```python
from build123d import *

# Parameters (mm, degrees)
EXTRUDE_1_DEPTH         = 8
SKETCH_3_OUTSIDE_W      = 189.666
SKETCH_3_OUTSIDE_H      = 189.666
SKETCH_3_OUTSIDE_R      = 12
CUT_EXTRUDE_1_DEPTH     = 41.024992192
CUT_EXTRUDE_1_DRAFT     = -60
HOLE_WIZARD_M30_1_D     = 26.5
HOLE_WIZARD_M30_1_DEPTH = 10
CHAMFER_1_SIZE          = 1
CHAMFER_2_SIZE          = 1


with BuildPart() as part:
    # 草图1 → 凸台-拉伸1 (new body)
    with BuildSketch(Plane.XY):
        Polygon((0, 13.856406461), (-12, 6.92820323), (-12, -6.92820323), (0, -13.856406461), (12, -6.92820323), (12, 6.92820323), align=None)
    extrude(amount=-EXTRUDE_1_DEPTH)

    # 草图2 → 旋转1 (revolve)
    with BuildSketch(Plane(origin=(0, 0, 0), x_dir=(0, 0, -1), z_dir=(1, 0, 0))):
        Polygon((8, 0), (8, 13.856406461), (11.143593539, 17), (32, 17), (32, 0), align=None)
    revolve(axis=Axis((0, 0, -32), (0, 0, 1)))


with BuildPart() as cut_extrude_1_tool:
    # 草图3 outside → 切除-拉伸1 (with draft: the straight prism first)
    with BuildSketch(Plane.XY):
        Rectangle(SKETCH_3_OUTSIDE_W, SKETCH_3_OUTSIDE_H)
        Circle(SKETCH_3_OUTSIDE_R, mode=Mode.SUBTRACT)
    extrude(amount=-CUT_EXTRUDE_1_DEPTH)
    # 切除-拉伸1: the draft: its side faces are tilted about the plane it starts from
    cut_extrude_1_sides = [cut_extrude_1_tool.faces().sort_by_distance(p)[0] for p in [
        (0, -94.833, -20.512496096),
        (94.833, 0, -20.512496096),
        (0, 94.833, -20.512496096),
        (-94.833, 0, -20.512496096),
        (-12, 0, -20.512496096),
    ]]
    draft(cut_extrude_1_sides, Plane.XY, CUT_EXTRUDE_1_DRAFT)


with BuildPart() as part_1:
    add(part.part)

    # 切除-拉伸1: cut by cut_extrude_1_tool
    add(cut_extrude_1_tool.part, mode=Mode.SUBTRACT)

    # 草图4 → 切除-旋转1 (revolve, cut)
    with BuildSketch(Plane(origin=(0, 0, 0), x_dir=(0, 0, -1), z_dir=(1, 0, 0)), mode=Mode.PRIVATE) as cut_revolve_1_sk:
        Polygon((0, 0), (0, -7), (6, -7), (6, -9), (14, -9), (14, -14), (15, -14), (15, -15), (22, -15), (22, 0), align=None)
    revolve(cut_revolve_1_sk.sketch.rotate(Axis((0, 0, -22), (0, 0, 1)), 270), axis=Axis((0, 0, -22), (0, 0, 1)), mode=Mode.SUBTRACT)

    # M30 螺纹孔1
    with Locations(Plane(origin=(0, 0, -32), x_dir=(-1, 0, 0), z_dir=(0, 0, -1))):
        with Locations((0, 0)):
            Hole(HOLE_WIZARD_M30_1_D / 2, depth=HOLE_WIZARD_M30_1_DEPTH)

    # 倒角1
    chamfer_1_edges = [part_1.edges().sort_by_distance(p)[0] for p in [
        (0, -17, -32),
    ]]
    chamfer(chamfer_1_edges, length=CHAMFER_1_SIZE)

    # 倒角2
    chamfer_2_edges = [part_1.edges().sort_by_distance(p)[0] for p in [
        (7, 0, 0),
        (9, 0, -14),
    ]]
    chamfer(chamfer_2_edges, length=CHAMFER_2_SIZE)


solid = part_1.part
```
Build history of the part. All positions in model axes, mm. A direction names the side the tool comes from. Coordinates: 2 decimals unless noted, no trailing zeros. Order: outer loops, then holes, each group sorted by start corner. A loop starts at its lowest first (then second) coordinate and runs counter-clockwise, first axis right, second up. Notation, with made-up numbers: M -16,77 L 17,77 A14 ccw 17,81 Z; hole C 30,-0.5 d4. An arc over 180 degrees is marked long. One line per question, with ' | ' between items. Start each with the question number.
1. Mould opens along X. For faces 4 (the face through (1.517, 6.834, -3.535)), 5 (the face through (10.76, -6.248, -0.256)), 6 (the face through (0.03, 12.443, -0.256)) say: +X half, -X half, draft (parallel to the pull), parting line (faces both ways), or undercut.
2. Cut at A-A (z = -21). Write the cut outline in (x, y), plus the area to 3 significant figures.
3. Wall check: line 1 along Y through (x, z) = (0, -3.1); line 2 along Y through (x, z) = (0, -14.45); line 3 along Z through (x, y) = (5.5, 11). Give the ranges that are in metal, low to high. Write a range as [from, to].
4. Tool access for faces 1 (the face through (-6, 11, -8)), 2 (the face through (-6.084, -10.344, -3.944)), 3 (the face through (5.92, -10.44, -3.94)): list every direction of +Z, -Z, +X, -X, +Y, -Y with a clear straight run to the whole face (end or side of a thin tool).
5. Cut at B-B (z = -8.5). Write the cut outline in (x, y), plus the area to 3 significant figures.
6. Flat gauge pins, fed straight in: P1, Ø8, axis at y = 3, z = -20, coming from the -X side; P2, Ø6, axis at y = 9.5, z = -23.5, coming from the +X side; P3, Ø5.5, axis at x = -2.5, y = 1.5, coming from the -Z side; P4, Ø16, axis at x = 0, y = 0, coming from the -Z side. Where does each tip first touch, or does it go through?
The answers:
1) face 4: undercut | face 5: +X half | face 6: parting line
2) outline: C 0,0 d34; hole C 0,0 d30 | area: 201 mm2
3) line 1: y = [-13.86, -7], [7, 13.86] | line 2: y = [-17, -14], [14, 17] | line 3: z = [-14, -8]
4) face 1: +Z, -X, +Y | face 2: +Z, -X, -Y | face 3: +Z, +X, -Y
5) outline: C 0,0 d28.71; hole C 0,0 d18 | area: 393 mm2
6) P1: stops at x = -17 | P2: stops at x = 15.71 | P3: passes through | P4: stops at z = -6
